Read the model definition and answer for the solid it produces. Units are mm, in the model's axes. A direction names the side the tool comes from. Coordinates: 2 decimals unless noted, no trailing zeros. Order: outer loops, then holes, each group sorted by start corner. A loop starts at its lowest first (then second) coordinate and runs counter-clockwise, first axis right, second up. Notation, with made-up numbers: (85, 63.5) -> (90, 63.5) arc R11 cw to (90, 81.5) -> close; hole circle Ø4 at (-5.5, -2.75). An arc over 180 degrees is marked (long way). Use CSV: the item, a comma, the result in double quotes.
```python
from build123d import *

# Parameters (mm, degrees)
SKETCH1_R           = 18
BOSS_EXTRUDE1_DEPTH = 2
SKETCH2_R           = 16
BOSS_EXTRUDE2_DEPTH = 1
SKETCH3_R           = 7.5
BOSS_EXTRUDE3_DEPTH = 2
FILLET2_R           = 1
SKETCH4_R           = 18
SKETCH4_R_2         = 17
CUT_EXTRUDE1_DEPTH  = 1
SKETCH5_R           = 15.789460751
SKETCH5_R_2         = 13.932235083
CUT_EXTRUDE2_DEPTH  = 1
SKETCH6_R           = 12.231632463
SKETCH6_R_2         = 3.890953776
CUT_EXTRUDE3_DEPTH  = 1
FILLET3_R           = 1
CHAMFER1_SIZE       = 7.115369722
CHAMFER1_SIZE_2     = 1


# Some blends are built 0.0001 mm under size
with BuildPart() as part:
    # Sketch1 → Boss-Extrude1 (new body)
    with BuildSketch(Plane.XY):
        Circle(SKETCH1_R)
    extrude(amount=BOSS_EXTRUDE1_DEPTH)

    # Sketch2 → Boss-Extrude2 (add)
    with BuildSketch(Plane.XY.offset(2)):
        Circle(SKETCH2_R)
    extrude(amount=BOSS_EXTRUDE2_DEPTH)

    # Sketch3 → Boss-Extrude3 (add)
    with BuildSketch(Plane.XY.offset(3)):
        Circle(SKETCH3_R)
    extrude(amount=BOSS_EXTRUDE3_DEPTH)

    # Fillet2
    fillet2_edges = [part.edges().sort_by_distance(p)[0] for p in [
        (-7.5, 0, 3),
        (-7.5, 0, 5),
        (-18, 0, 2),
        (-16, 0, 3),
    ]]
    fillet(fillet2_edges, radius=FILLET2_R - 0.0001)  # a hair under: the kernel refuses the full size

    # Sketch4 → Cut-Extrude1 (cut)
    with BuildSketch(Plane(origin=(0, 0, 0), x_dir=(-1, 0, 0), z_dir=(0, 0, -1))):
        Circle(SKETCH4_R)
        Circle(SKETCH4_R_2, mode=Mode.SUBTRACT)
    extrude(amount=-CUT_EXTRUDE1_DEPTH, mode=Mode.SUBTRACT)

    # Sketch5 → Cut-Extrude2 (cut)
    with BuildSketch(Plane(origin=(0, 0, 0), x_dir=(-1, 0, 0), z_dir=(0, 0, -1))):
        Circle(SKETCH5_R)
        Circle(SKETCH5_R_2, mode=Mode.SUBTRACT)
    extrude(amount=-CUT_EXTRUDE2_DEPTH, mode=Mode.SUBTRACT)

    # Sketch6 → Cut-Extrude3 (cut)
    with BuildSketch(Plane(origin=(0, 0, 0), x_dir=(-1, 0, 0), z_dir=(0, 0, -1))):
        Circle(SKETCH6_R)
        Circle(SKETCH6_R_2, mode=Mode.SUBTRACT)
    extrude(amount=-CUT_EXTRUDE3_DEPTH, mode=Mode.SUBTRACT)

    # Fillet3
    fillet3_edges = [part.edges().sort_by_distance(p)[0] for p in [
        (3.890953776, 0, 0),
    ]]
    fillet(fillet3_edges, radius=FILLET3_R - 0.0001)  # a hair under: the kernel refuses the full size

    # Chamfer1
    # the kernel refuses this chamfer: 7.115369722, 1 mm, written as the material it adds along each edge
    with BuildSketch(Plane(origin=(0, 0, 1), x_dir=(-1, 0, 0), z_dir=(0, -1, 0))) as chamfer1_piece_1_section:
        Polygon((12.231632463 - CHAMFER1_SIZE, 0), (12.231632463, CHAMFER1_SIZE_2), (12.231632463, 0), align=None)
    chamfer1_piece_1 = revolve(axis=Axis((0, 0, 1), (0, 0, -1)), mode=Mode.PRIVATE)
    chamfer1_piece_1 = split(chamfer1_piece_1, bisect_by=Plane(origin=(8.54226682, 0, 0), z_dir=(0, 0, 1)), keep=Keep.TOP, mode=Mode.PRIVATE)
    add(chamfer1_piece_1)


solid = part.part
```
Item 1: Find section A-A, the plane z = 3.55. Give the vertices of the cut face in (x, y).
Return value:
outline,"circle Ø15.21 at (0, 0)"
Item 2: Each of these flat-tipped pins is pushed along its axis until it touches: P1, Ø1, axis at x = 12, y = 10.5, coming from the +Z side; P2, Ø4, axis at x = -6, y = 5, coming from the -Z side. Where does it stop, or does it pass through?
Return value:
P1,"stops at z = 2.9"
P2,"stops at z = 0.34"
Item 3: The mould has two halves that part along Y. Classify faces 4 (the cylindrical face through (-9.139, 14.334, 0.493)), 5 (the flat face through (1, 4, 1)), 6 (the flat face through (0, 0, 5)): +Y half, -Y half, draft (parallel to the pull), parting line (faces both ways), or undercut.
Return value:
face 4,"parting line"
face 5,"undercut"
face 6,"draft"
Item 4: Straight lines are drawn through the part: line 1 along Z through (x, y) = (-2.5, 4.5); line 2 along Z through (x, y) = (-15.5, -5); line 3 along X through (y, z) = (14, 1.7). For each, find the intervals that lie inside material, in ascending order.
Return value:
line 1,"z = 1 to 5"
line 2,"z = 0 to 2"
line 3,"x = -10.85 to 10.85"
Item 5: A tool of negligible diameter and unlimited length cuts with its end or side. For faces 1 (the flat face through (11.3, -11.3, 0)), 2 (the flat face through (13, -10, 2)), 3 (the flat face through (-6, -13, 1)), from which of +Z, -Z, +X, -X, +Y, -Y can it reach the whole face along a straight path? Write none if from no direction.
Return value:
face 1,"-Z, +X, -X, +Y, -Y"
face 2,"+Z"
face 3,"-Z"
